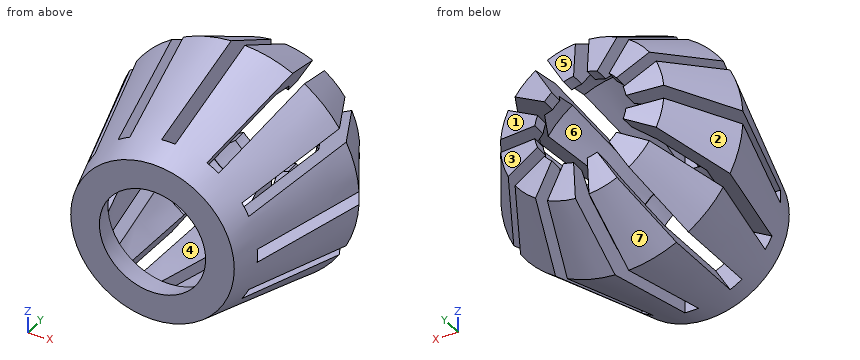
from build123d import *

# Parameters (mm, degrees)
SKETCH_6_R               = 6.75
CUT_EXTRUDE_3_DEPTH      = 2.049864
CUT_EXTRUDE_3_DEPTH_BACK = 32.547005
SKETCH_8_W               = 2
SKETCH_8_H               = 35.547006
SKETCH_8_W_2             = 35.547006
SKETCH_8_H_2             = 2
CUT_EXTRUDE_4_DEPTH      = 1.459315
CUT_EXTRUDE_4_DEPTH_BACK = 27.547005


with BuildPart() as part:
    # 草图2 → 旋转1 (revolve)
    with BuildSketch(Plane.XY):
        Polygon((0, 11.049864), (0, 10), (-12, 10), align=None)
        Polygon((0, 10), (0, -21.547005), (-12, -21.547005), (-17.773503, 0), (-12, 10), align=None)
    revolve(axis=Axis((0, -736.81226, 0), (0, 1, 0)))

    # 草图7 one side → 切除-旋转2 (revolve, cut)
    with BuildSketch(Plane.XY):
        Polygon((0, -17.547005), (0, 7.034585), (-9.577032, 6.196703), (-13.480974, -0.565122), (-8.930692, -17.547005), align=None)
    revolve(axis=Axis((0, -1000, 0), (0, 1, 0)), mode=Mode.SUBTRACT)

    # 草图6 → 切除-拉伸3 (cut, two sides)
    with BuildSketch(Plane(origin=(0, 10, 0), x_dir=(1, 0, 0), z_dir=(0, 1, 0))) as cut_extrude_3_sk:
        Circle(SKETCH_6_R)
    extrude(amount=CUT_EXTRUDE_3_DEPTH, mode=Mode.SUBTRACT)
    extrude(cut_extrude_3_sk.sketch, amount=-CUT_EXTRUDE_3_DEPTH_BACK, mode=Mode.SUBTRACT)

    # 草图8 → 切除-拉伸4 (cut, two sides)
    with BuildSketch(Plane(origin=(0, 10, 0), x_dir=(1, 0, 0), z_dir=(0, 1, 0))) as cut_extrude_4_sk:
        Polygon((9.752777, 14.892305), (-8.020726, -15.892305), (-9.752777, -14.892305), (8.020726, 15.892305), align=None)
        Rectangle(SKETCH_8_W, SKETCH_8_H)
        Polygon((15.892305, 8.020726), (-14.892305, -9.752777), (-15.892305, -8.020726), (14.892305, 9.752777), align=None)
        Rectangle(SKETCH_8_W_2, SKETCH_8_H_2)
        Polygon((14.892305, -9.752777), (-15.892305, 8.020726), (-14.892305, 9.752777), (15.892305, -8.020726), align=None)
        Polygon((8.020726, -15.892305), (-9.752777, 14.892305), (-8.020726, 15.892305), (9.752777, -14.892305), align=None)
    extrude(amount=CUT_EXTRUDE_4_DEPTH, mode=Mode.SUBTRACT)
    extrude(cut_extrude_4_sk.sketch, amount=-CUT_EXTRUDE_4_DEPTH_BACK, mode=Mode.SUBTRACT)

    # 草图10 → 切除-旋转3 (revolve, cut)
    with BuildSketch(Plane.XY):
        with BuildLine():
            Line((6.675515, 8.459315), (6.675515, 6.444036))
            add(Edge.make_bspline(
                [(9.524681, 6.196703), (8.574975, 6.279337), (7.625259, 6.361861), (6.675515, 6.444036)],
                knots=[0, 0, 0, 0, 1, 1, 1, 1], degree=3))
            Line((9.524681, 6.196703), (6.675515, 8.459315))
        make_face()
    revolve(axis=Axis((0, -1000, 0), (0, 1, 0)), mode=Mode.SUBTRACT)

    # 草图11 → 切除-旋转4 (revolve, cut)
    with BuildSketch(Plane.XY):
        Polygon((6.75, -21.547005), (6.75, -17.547005), (8.874529, -17.547005), (7.795949, -21.547005), align=None)
    revolve(axis=Axis((0, -1000, 0), (0, 1, 0)), mode=Mode.SUBTRACT)


solid = part.part
Work out the finished part from the listing and answer in its coordinate system (mm). Face numbers are marked on the shaded views. A direction names the side the tool comes from. Give positions to 0.01 mm unless a question says otherwise; leave off trailing zeros. Order: outer loops, then holes, each group sorted by start corner. A loop starts at its lowest first (then second) coordinate and runs counter-clockwise, first axis right, second up. Notation, with made-up numbers: (-29, 61) -> (8, 61) arc R34 cw to (8, 100) -> close; hole circle Ø7 at (64, -9). An arc over 180 degrees is marked (long way). One line per item, written item: value.
Item 1: A tool of negligible diameter and unlimited length cuts with its end or side. For the marked faces 1, 2, 3 and 4, from which of +Z, -Z, +X, -X, +Y, -Y can it reach the whole face along a straight path? Write none if from no direction.
Answer sheet:
face 1: +Z, +X, +Y
face 2: -Z, -X, +Y
face 3: -Z, +X, +Y
face 4: none
Item 2: Find section C-C, the plane y = -13. State how many separate pieces and enclosed holes the cut face has, plus the area to 3 significant figures.
Answer sheet:
separate pieces: 12
enclosed holes: 0
area: 218 mm²
Item 3: Find section A-A, the plane z = 0. Give the vertices of the cut face in (x, y), plus the area to 3 significant figures.
Answer sheet:
outline: (-13.07, -17.55) -> (-12, -21.55) -> (-7.8, -21.55) -> (-8.87, -17.55) -> close; (7.8, -21.55) -> (12, -21.55) -> (13.07, -17.55) -> (8.87, -17.55) -> close
area: 33.6 mm²
Item 4: Determine the mould class of the marked faces 5, 6 and 7 for opening direction Z: released by +Z, released by -Z, zero draft, split by the parting line, or undercut.
Answer sheet:
face 5: released by +Z
face 6: undercut
face 7: released by -Z
Item 5: Flat-ended cylindrical pins translate along their axes: P1, Ø5.5, axis at y = -1, z = 12.5, coming from the -X side; P2, Ø3.5, axis at x = 12.5, y = -0.5, coming from the +Z side; P3, Ø3.5, axis at x = 12.5, y = 3.5, coming from the -Z side. Find the tip coordinate at first contact, or state that the pin passes through.
Answer sheet:
P1: x = -14.74
P2: z = 14.1
P3: z = -12.02
Item 6: Find section B-B, the plane x = 0. Give the vertices of the cut face in (y, z).
Answer sheet:
outline: (-21.55, -12) -> (-17.55, -13.07) -> (-17.55, -8.87) -> (-21.55, -7.8) -> close; (-21.55, 7.8) -> (-17.55, 8.87) -> (-17.55, 13.07) -> (-21.55, 12) -> close
Item 7: Straight lines are drawn through the part: probe 1 along Z at (x, y) = (-11.5, -11); probe 2 along X at (y, z) = (-16, 7); probe 3 along X at (y, z) = (4.5, 3). For each, find the intervals that lie inside material, in ascending order.
Answer sheet:
probe 1: -9.36 to -7.79, -5.48 to -1, 1 to 5.48, 7.79 to 9.36
probe 2: -10.12 to -6.19, 6.19 to 10.12
probe 3: -14.88 to -10.12, 10.12 to 14.88
